Could you check a few things on this drawing? It's one solid part, dimensions in mm from its lowest x, y, z. A direction names the side the tool comes from. Give positions to 0.01 mm unless a question says otherwise; leave off trailing zeros. Loops run counter-clockwise (first coordinate to the right, second up) from the corner with the lowest first, then second, coordinate; pieces in that order, holes last. Notation, with made-up numbers: M 31.25,77.25 L 90.25,77.25 A32 cw 90.25,111.25 Z; hole C 74,78.5 d1. An arc over 180 degrees is marked long. Return JSON: item names as keys, results as strings. Group by question number.
1. For the marked faces 5, 6 and 7, which set-ups out of +Z, -Z, +X, -X, +Y, -Y let a thin tool reach every point of the face, with its end or its side?
2. If we section it at B-B (z = 7.5): Write out the boundary of the cut face in (x, y), plus the area to 3 significant figures.
3. If we section it at A-A (y = 37): Write out the boundary of the cut face in (x, z).
4. If we mould it in two halves opening along X, with no side actions, what happens to the marked faces 1, 2, 3 and 4? For each: +X half, -X half, draft (parallel to the pull), parting line (faces both ways), or undercut.
5. For pin 1 (8 mm diameter, centred on x = 35, z = 71.5, fed in from -Y); pin 2 (12.5 mm diameter, centred on x = 95, z = 51, fed in from -Y), each with a flat end and sliding along its axis, tell me the tip position at first contact or that it passes through.
6. Please list where these lines run through material, in increasing order: line 1 (Y direction, x = 59, z = 62); line 2 (Y direction, x = 60, z = 8.5); line 3 (Y direction, x = 12.5, z = 40).
7. If we section it at C-C (x = 61): Write out the boundary of the cut face in (y, z), plus the area to 3 significant figures.
8. If we section it at D-D (z = 79): Write out the boundary of the cut face in (x, y), plus the area to 3 significant figures.
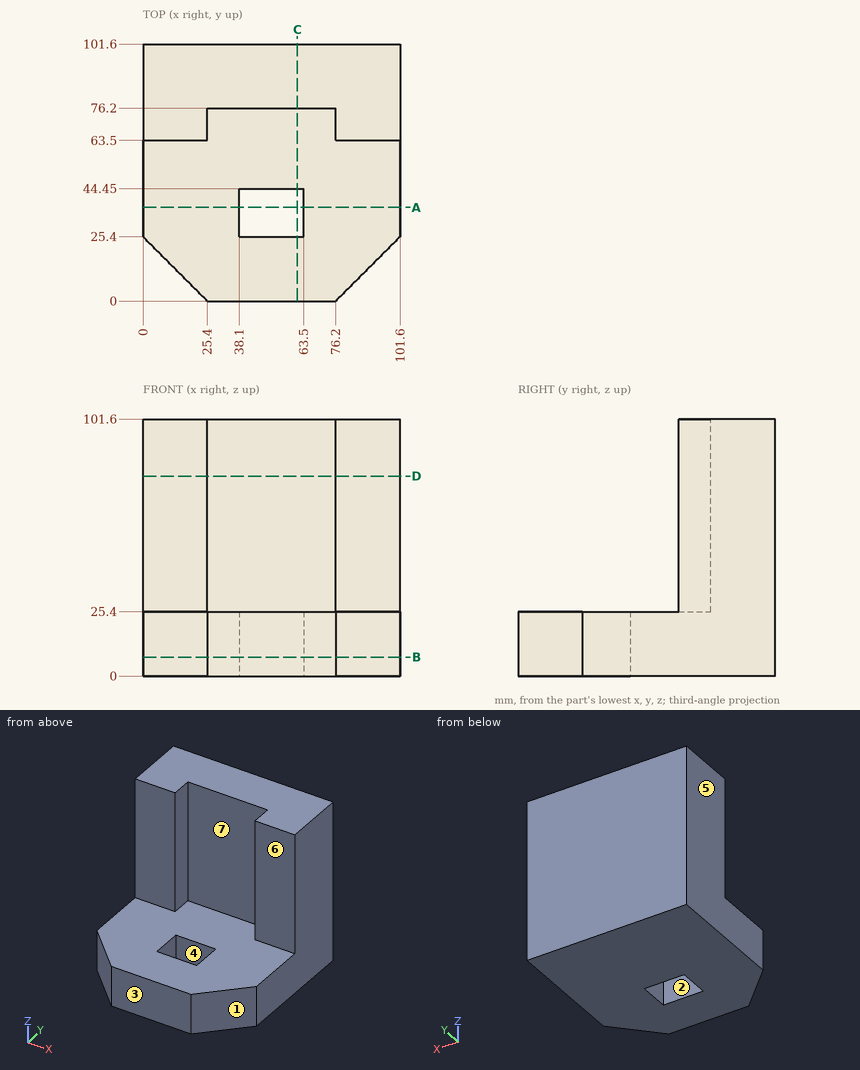
Answer:
{
 "1": {"face 5": "+Z, -Z, -X, +Y, -Y", "face 6": "+Z, +X, -X, -Y", "face 7": "+Z, -Y"},
 "2": {"outline": "M 0,25.4 L 25.4,0 L 76.2,0 L 101.6,25.4 L 101.6,101.6 L 0,101.6 Z; hole M 38.1,25.4 L 63.5,25.4 L 63.5,44.45 L 38.1,44.45 Z", "area": "9,190 mm²"},
 "3": {"outline": "M 0,0 L 38.1,0 L 38.1,25.4 L 0,25.4 Z; M 63.5,0 L 101.6,0 L 101.6,25.4 L 63.5,25.4 Z"},
 "4": {"face 1": "+X half", "face 2": "undercut", "face 3": "draft", "face 4": "undercut"},
 "5": {"pin 1": "stops at y = 76.2", "pin 2": "stops at y = 63.5"},
 "6": {"line 1": "y = 76.2 to 101.6", "line 2": "y = 0 to 25.4, 44.45 to 101.6", "line 3": "y = 63.5 to 101.6"},
 "7": {"outline": "M 0,0 L 25.4,0 L 25.4,25.4 L 0,25.4 Z; M 44.45,0 L 101.6,0 L 101.6,101.6 L 76.2,101.6 L 76.2,25.4 L 44.45,25.4 Z", "area": "4,030 mm²"},
 "8": {"outline": "M 0,63.5 L 25.4,63.5 L 25.4,76.2 L 76.2,76.2 L 76.2,63.5 L 101.6,63.5 L 101.6,101.6 L 0,101.6 Z", "area": "3,230 mm²"}
}
